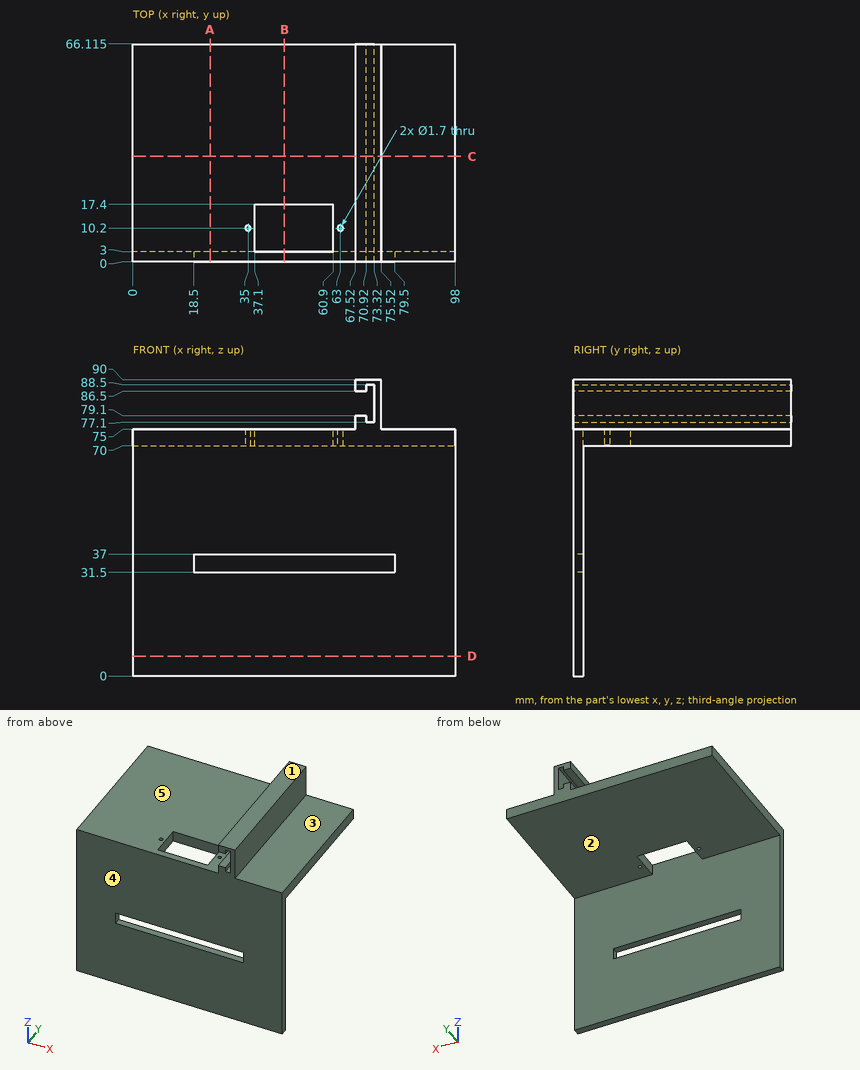
Job drawing, mm, ordinate dimensions from the low corner. One solid piece. A direction names the side the tool comes from. Give positions to 0.01 mm unless a question says otherwise; leave off trailing zeros. Write each loop counter-clockwise with the first axis right and the second up, starting at its lowest first coordinate (ties: lowest second). Pieces come first, ordered by that corner, then holes. Notation, with made-up numbers: (39, 30) - (45, 30) arc R31 ccw to (45, 55) - close; hole circle Ø4 at (-24.75, 55.25). An arc over 180 degrees is marked (long way). Use one line per item in the form item = value. Start each with the question number.
1. Band-saw the part on B-B on x = 46. Write the cut outline in (y, z) (1 decimal).
2. Band-saw the part on C-C on y = 32. Write the cut outline in (x, z).
3. Probe line 1 (Y direction, x = 73.5, z = 13); line 2 (Z direction, x = 63, y = 11.5); line 3 (Z direction, x = 74, y = 50.5). List the from-to ranges inside material, lowest first. Write a range as [from, to].
4. 3-axis set-ups, long thin cutter, end or side, ignore diameter. For the marked faces 1, 2, 3, 4 and 5: which of +Z, -Z, +X, -X, +Y, -Y reach the whole face in a straight line?
5. Band-saw the part on D-D on z = 6. Write the cut outline in (x, y), plus the area to 3 significant figures.
6. Band-saw the part on A-A on x = 23.5. Write the cut outline in (y, z) (1 decimal), plus the area to 3 significant figures.
7. Drop flat-ended pins along their axis: pin 1 Ø3 at (y, z) = (25.5, 89) entering from -X; pin 2 Ø2.5 at (x, y) = (50, 1.5) entering from +Z; pin 3 Ø2.5 at (x, y) = (69.5, 29.5) entering from -Z; pin 4 Ø6 at (x, z) = (24.5, 41) entering from -Y. Give the stop position or say it passes through.
Conclusion:
q1.outline = (0, 0) - (3, 0) - (3, 31.5) - (0, 31.5) - close; (0, 37) - (3, 37) - (3, 75) - (0, 75) - close; (17.4, 70) - (66.1, 70) - (66.1, 75) - (17.4, 75) - close
q2.outline = (0, 70) - (98, 70) - (98, 75) - (75.52, 75) - (75.52, 90) - (67.52, 90) - (67.52, 86.5) - (70.92, 86.5) - (70.92, 88.5) - (73.32, 88.5) - (73.32, 77.1) - (70.92, 77.1) - (70.92, 79.1) - (67.52, 79.1) - (67.52, 75) - (0, 75) - close
q3.line_1 = [0, 3]
q3.line_2 = [70, 75]
q3.line_3 = [70, 90]
q4.face_1 = +Z, +X, -X, +Y, -Y
q4.face_2 = -Z, +X, -X, +Y
q4.face_3 = +Z, +X, +Y, -Y
q4.face_4 = +Z, -Z, +X, -X, -Y
q4.face_5 = +Z, -X, +Y, -Y
q5.outline = (0, 0) - (98, 0) - (98, 3) - (0, 3) - close
q5.area = 294 mm²
q6.outline = (0, 0) - (3, 0) - (3, 31.5) - (0, 31.5) - close; (0, 37) - (3, 37) - (3, 70) - (66.1, 70) - (66.1, 75) - (0, 75) - close
q6.area = 524 mm²
q7.pin_1 = 67.52
q7.pin_2 = 75
q7.pin_3 = 70
q7.pin_4 = 0
